from build123d import *

# Parameters (mm, degrees)
RESSALTO_EXTRUS_O1_DEPTH = 4


with BuildPart() as part:
    # Esboço1 → Ressalto-extrusão1 (new body)
    with BuildSketch(Plane.XY):
        with BuildLine():
            Line((20.408082875, 0.8), (33.077498183, 0.8))
            Line((33.077498183, 0.8), (33.908082875, 0.8))
            ThreePointArc((33.908082875, 0.8), (35.05690323, -1.973497683), (32.283405548, -0.824677327))
            Line((32.283405548, -0.824677327), (32.083405548, -0.824677327))
            ThreePointArc((32.083405548, -0.824677327), (35.198324587, -2.114919039), (33.908082875, 1))
            Line((33.908082875, 1), (20.408082875, 1))
            Line((20.408082875, 1), (20.408082875, 0.8))
        make_face()
    extrude(amount=RESSALTO_EXTRUS_O1_DEPTH)


solid = part.part
Check sheet for the modelled part. Datum: model origin and axes. Units: mm. Give positions to 0.01 mm unless a question says otherwise; leave off trailing zeros. Order: outer loops, then holes, each group sorted by start corner. A loop starts at its lowest first (then second) coordinate and runs counter-clockwise, first axis right, second up. Notation, with made-up numbers: (-13, -27) - (19, -27) arc R30 ccw to (19, 4) - close; hole circle Ø10 at (6, 88). An arc over 180 degrees is marked (long way). Answer as CSV lines item,"result".
1. Section check C-C (x = 26). Record the boundary of the cut face in (y, z).
Result sheet:
outline,"(0.8, 0) - (1, 0) - (1, 4) - (0.8, 4) - close"
2. Section check B-B (z = 1.75). Record the boundary of the cut face in (x, y), then the cut area to 3 significant figures.
Result sheet:
outline,"(20.41, 0.8) - (33.91, 0.8) arc R1.62 cw (long way) to (32.28, -0.82) - (32.08, -0.82) arc R1.82 ccw (long way) to (33.91, 1) - (20.41, 1) - close"
area,"4.33 mm²"
3. Go/stop test with flat-tipped pins: P1, Ø2, axis at x = 24, z = 3, coming from the -Y side; P2, Ø1.5, axis at x = 30.5, y = 0.5, coming from the +Z side. Record where each tip stops, or that it passes through.
Result sheet:
P1,"y = 0.8"
P2,"z = 4"
4. Mould release check, pull along Y, two halves, no side actions. Record for faces 1 (the face through (27, 1, 2)), 2 (the face through (35.155, -2.157, 1.972)), 3 (the face through (35.094, -1.935, 1.972)): released by +Y, released by -Y, zero draft, split by the parting line, or undercut.
Result sheet:
face 1,"released by +Y"
face 2,"split by the parting line"
face 3,"undercut"
5. Section check A-A (y = -1.4). Record the boundary of the cut face in (x, z), then the cut area to 3 significant figures.
Result sheet:
outline,"(32.18, 0) - (32.39, 0) - (32.39, 4) - (32.18, 4) - close; (35.43, 0) - (35.64, 0) - (35.64, 4) - (35.43, 4) - close"
area,"1.70 mm²"
6. Section check D-D (y = 0.2). Record the boundary of the cut face in (x, z).
Result sheet:
outline,"(35.17, 0) - (35.42, 0) - (35.42, 4) - (35.17, 4) - close"
7. Scan lines: probe 1 along Y at (x, z) = (30.5, 0.7); probe 2 along X at (y, z) = (-1.05, 3.6); probe 3 along X at (y, z) = (-1.65, 2.75). Record each from-to range of solid material in increasing order. Write a range as from..to.
Result sheet:
probe 1,"0.8..1"
probe 2,"32.1..32.3, 35.52..35.72"
probe 3,"32.28..32.51, 35.31..35.54"
